from build123d import *

# Parameters (mm, degrees)
SKETCH1_R           = 2.1
BOSS_EXTRUDE1_DEPTH = 500


with BuildPart() as part:
    # Sketch1 → Boss-Extrude1 (new body)
    with BuildSketch(Plane.XY):
        with BuildLine():
            Line((3.69, 0), (3.9, -0.21))
            Line((3.9, -0.21), (3.9, -2.839339828))
            Line((3.9, -2.839339828), (6.560660172, -5.5))
            Line((6.560660172, -5.5), (8.2, -5.5))
            Line((8.2, -5.5), (8.2, -3.125))
            Line((8.2, -3.125), (8.545, -3.125))
            Line((8.545, -3.125), (10, -4.58))
            Line((10, -4.58), (10, -15.42))
            Line((10, -15.42), (8.545, -16.875))
            Line((8.545, -16.875), (8.2, -16.875))
            Line((8.2, -16.875), (8.2, -14.5))
            Line((8.2, -14.5), (6.560660172, -14.5))
            Line((6.560660172, -14.5), (3.9, -17.160660172))
            Line((3.9, -17.160660172), (3.9, -19.79))
            Line((3.9, -19.79), (3.69, -20))
            Line((3.69, -20), (3.9, -20.21))
            Line((3.9, -20.21), (3.9, -22.839339828))
            Line((3.9, -22.839339828), (6.560660172, -25.5))
            Line((6.560660172, -25.5), (8.2, -25.5))
            Line((8.2, -25.5), (8.2, -23.125))
            Line((8.2, -23.125), (8.545, -23.125))
            Line((8.545, -23.125), (10, -24.58))
            Line((10, -24.58), (10, -29.5))
            ThreePointArc((10, -29.5), (9.853553391, -29.853553391), (9.5, -30))
            Line((9.5, -30), (4.58, -30))
            Line((4.58, -30), (3.125, -28.545))
            Line((3.125, -28.545), (3.125, -28.2))
            Line((3.125, -28.2), (5.5, -28.2))
            Line((5.5, -28.2), (5.5, -26.560660172))
            Line((5.5, -26.560660172), (2.839339828, -23.9))
            Line((2.839339828, -23.9), (0.21, -23.9))
            Line((0.21, -23.9), (0, -23.69))
            Line((0, -23.69), (-0.21, -23.9))
            Line((-0.21, -23.9), (-2.839339828, -23.9))
            Line((-2.839339828, -23.9), (-5.5, -26.560660172))
            Line((-5.5, -26.560660172), (-5.5, -28.2))
            Line((-5.5, -28.2), (-3.125, -28.2))
            Line((-3.125, -28.2), (-3.125, -28.545))
            Line((-3.125, -28.545), (-4.58, -30))
            Line((-4.58, -30), (-9.5, -30))
            ThreePointArc((-9.5, -30), (-9.853553391, -29.853553391), (-10, -29.5))
            Line((-10, -29.5), (-10, -24.58))
            Line((-10, -24.58), (-8.545, -23.125))
            Line((-8.545, -23.125), (-8.2, -23.125))
            Line((-8.2, -23.125), (-8.2, -25.5))
            Line((-8.2, -25.5), (-6.560660172, -25.5))
            Line((-6.560660172, -25.5), (-3.9, -22.839339828))
            Line((-3.9, -22.839339828), (-3.9, -20.21))
            Line((-3.9, -20.21), (-3.69, -20))
            Line((-3.69, -20), (-3.9, -19.79))
            Line((-3.9, -19.79), (-3.9, -17.160660172))
            Line((-3.9, -17.160660172), (-6.560660172, -14.5))
            Line((-6.560660172, -14.5), (-8.2, -14.5))
            Line((-8.2, -14.5), (-8.2, -16.875))
            Line((-8.2, -16.875), (-8.545, -16.875))
            Line((-8.545, -16.875), (-10, -15.42))
            Line((-10, -15.42), (-10, -4.58))
            Line((-10, -4.58), (-8.545, -3.125))
            Line((-8.545, -3.125), (-8.2, -3.125))
            Line((-8.2, -3.125), (-8.2, -5.5))
            Line((-8.2, -5.5), (-6.560660172, -5.5))
            Line((-6.560660172, -5.5), (-3.9, -2.839339828))
            Line((-3.9, -2.839339828), (-3.9, -0.21))
            Line((-3.9, -0.21), (-3.69, 0))
            Line((-3.69, 0), (-3.9, 0.21))
            Line((-3.9, 0.21), (-3.9, 2.839339828))
            Line((-3.9, 2.839339828), (-6.560660172, 5.5))
            Line((-6.560660172, 5.5), (-8.2, 5.5))
            Line((-8.2, 5.5), (-8.2, 3.125))
            Line((-8.2, 3.125), (-8.545, 3.125))
            Line((-8.545, 3.125), (-10, 4.58))
            Line((-10, 4.58), (-10, 9.5))
            ThreePointArc((-10, 9.5), (-9.853553391, 9.853553391), (-9.5, 10))
            Line((-9.5, 10), (-4.58, 10))
            Line((-4.58, 10), (-3.125, 8.545))
            Line((-3.125, 8.545), (-3.125, 8.2))
            Line((-3.125, 8.2), (-5.5, 8.2))
            Line((-5.5, 8.2), (-5.5, 6.560660172))
            Line((-5.5, 6.560660172), (-2.839339828, 3.9))
            Line((-2.839339828, 3.9), (-0.21, 3.9))
            Line((-0.21, 3.9), (0, 3.69))
            Line((0, 3.69), (0.21, 3.9))
            Line((0.21, 3.9), (2.839339828, 3.9))
            Line((2.839339828, 3.9), (5.5, 6.560660172))
            Line((5.5, 6.560660172), (5.5, 8.2))
            Line((5.5, 8.2), (3.125, 8.2))
            Line((3.125, 8.2), (3.125, 8.545))
            Line((3.125, 8.545), (4.58, 10))
            Line((4.58, 10), (9.5, 10))
            ThreePointArc((9.5, 10), (9.853553391, 9.853553391), (10, 9.5))
            Line((10, 9.5), (10, 4.58))
            Line((10, 4.58), (8.545, 3.125))
            Line((8.545, 3.125), (8.2, 3.125))
            Line((8.2, 3.125), (8.2, 5.5))
            Line((8.2, 5.5), (6.560660172, 5.5))
            Line((6.560660172, 5.5), (3.9, 2.839339828))
            Line((3.9, 2.839339828), (3.9, 0.21))
            Line((3.9, 0.21), (3.69, 0))
        make_face()
        with Locations((0, -20)):
            Circle(SKETCH1_R, mode=Mode.SUBTRACT)
        Circle(SKETCH1_R, mode=Mode.SUBTRACT)
        Polygon((-8.2, -12.7), (-6.239339828, -12.7), (-2.839339828, -16.1), (2.839339828, -16.1), (6.239339828, -12.7), (8.2, -12.7), (8.2, -7.3), (6.239339828, -7.3), (2.839339828, -3.9), (-2.839339828, -3.9), (-6.239339828, -7.3), (-8.2, -7.3), align=None, mode=Mode.SUBTRACT)
    extrude(amount=BOSS_EXTRUDE1_DEPTH)


solid = part.part
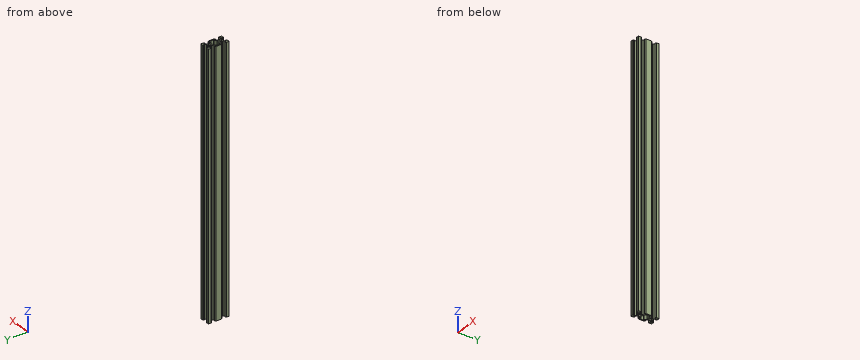
For this review, take the finished solid that the model builds, in its own axes (mm). Give positions to 0.01 mm unless a question says otherwise; leave off trailing zeros. Put each result on its own line as item: value. Start each with the question number.
(1) Add section A-A, the plane z = 449. Give the number of separate pieces and of enclosed holes in the cut face, then the cut area to 3 significant figures.
(2) For pin 1 (0.7 mm diameter, centred on y = -4, z = 260, fed in from +X); pin 2 (1.7 mm diameter, centred on x = 0.5, z = 134, fed in from -Y); pin 3 (1.7 mm diameter, centred on x = -1, z = 345.5, fed in from +Y), all flat-tipped, find the tip position at first contact; note any pin that passes through.
(3) Wall thickness on L1, parallel to Y at x = 0, z = 294.5; L2, parallel to Y at x = -6.5, z = 255; L3, parallel to X at y = -9.5, z = 447: over which ranges is each line inside the solid? List them lowest first.
Result:
1. separate pieces: 1
1. enclosed holes: 3
1. area: 300 mm^2
2. pin 1: stops at x = 9.77
2. pin 2: stops at y = -23.9
2. pin 3: stops at y = 3.9
3. L1: y = -23.69 to -22.1, -17.9 to -16.1, -3.9 to -2.1, 2.1 to 3.69
3. L2: y = -30 to -25.44, -14.56 to -12.7, -7.3 to -5.44, 5.44 to 10
3. L3: x = -10 to -8.2, 8.2 to 10
